Part model, mm, in its own coordinate system. A direction names the side the tool comes from. Give positions to 0.01 mm unless a question says otherwise; leave off trailing zeros. Write each loop counter-clockwise with the first axis right and the second up, starting at its lowest first coordinate (ties: lowest second). Pieces come first, ordered by that corner, then holes. Notation, with made-up numbers: M 74,-5.5 L 109,-5.5 A17 ccw 109,6.5 Z; hole C -11.5,-16 d6. An arc over 180 degrees is marked long. Use CSV: the item, a comma, the result in double quotes. Start each with the question number.
Item 1: Cut at B-B (z = 7). List the corners of the cut face in (x, y), then the cut area to 3 significant figures.
Item 2: Which spindle directions (+Z, -Z, +X, -X, +Y, -Y) get a long thin tool onto all of the face, cutting with end or side? Do faces 1 (the flat face through (0.8, 0, 0)), 2 (the flat face through (7, 0, 2.5)), 3 (the flat face through (5, -16, 2)), 4 (the cylindrical face through (5.042, 5.285, -0.051)), 5 (the cylindrical face through (1.877, 0.088, 0.528)). Say none if no direction does.
Item 3: Pin check, flat tips, straight feed: pin 1 (1.2 mm diameter, centred on x = 4.5, y = -8, fed in from -Z); pin 2 (0.6 mm diameter, centred on y = -13.5, z = 0, fed in from +X); pin 3 (1.2 mm diameter, centred on x = 3, y = 0.5, fed in from +Z). Stop position of each tip, or through.
Item 4: Cut at A-A (y = -21). List the corners of the cut face in (x, z), then the cut area to 3 significant figures.
Item 5: Cut at C-C (y = 0). List the corners of the cut face in (x, z) (3 decimals), then the cut area to 3 significant figures.
Item 6: Drill centre lines: line 1 (Z direction, x = 1.5, y = -10.5); line 2 (Y direction, x = 2, z = 5.25); line 3 (Y direction, x = 5, z = 0.5). Where is each one in solid material? Low to high. Write a range as [from, to].
Item 7: Cut at D-D (z = 3.5). List the corners of the cut face in (x, y), then the cut area to 3 significant figures.
Item 8: Mould opens along Y. For faces 6 (the flat face through (6, -15, 2)), 7 (the flat face through (2, 0, -2.5)), 8 (the flat face through (4.6, 16.4, 0.55)), 9 (the cylindrical face through (5.042, -4.699, -2.215)) say: released by +Y, released by -Y, zero draft, split by the parting line, or undercut.
from build123d import *

# Parameters (mm, degrees)
F0_W      = 58
F0_H      = 5
F1_DEPTH  = 2
F2_W      = 13
F2_H      = 0.5
F3_DEPTH  = 0.8
F4_W      = 58
F4_H      = 2.25
F5_DEPTH  = 6
F6_W      = 6
F6_H      = 10
F7_DEPTH  = 2.75
F8_R      = 2
F9_DEPTH  = 4
F10_R     = 1
F12_DEPTH = 4
F13_W     = 22
F13_H     = 5
F14_DEPTH = 0.8
F15_R     = 0.5
F16_W     = 6.8
F16_H     = 13
F17_DEPTH = 0.3
F18_W     = 3
F18_H     = 3
F19_DEPTH = 1.95


# Not quite as in the source:
# - a pattern or mirror of a feature is missing from the dataset's text; its kind, count and spacing are read off the source's solid


with BuildPart() as f1:
    # F0 (on Right) → F1 (new body)
    with BuildSketch(Plane.YZ):
        Rectangle(F0_W, F0_H)
    extrude(amount=F1_DEPTH)

    # F2 (on face) → F3 (cut)
    with BuildSketch(Plane.YZ.offset(2)):
        with Locations((16.5, 0)):
            Rectangle(F2_W, F2_H)
        with Locations((-16.5, 0)):
            Rectangle(F2_W, F2_H)
    extrude(amount=-F3_DEPTH, mode=Mode.SUBTRACT)

    # F4 (on face) → F5 (join)
    with BuildSketch(Plane.YZ.offset(2)):
        with Locations((0, 1.375)):
            Rectangle(F4_W, F4_H)
    extrude(amount=F5_DEPTH)

    # F6 (on face) → F7 (join, through all)
    with BuildSketch(Plane(origin=(0, 0, 0.25), x_dir=(1, 0, 0), z_dir=(0, 0, -1))):
        with Locations((5, 0)):
            Rectangle(F6_W, F6_H)
    extrude(amount=F7_DEPTH)

    # F8 (on face) → F9 (cut)
    with BuildSketch(Plane.XY.offset(2.5)):
        with Locations((3.875, 0)):
            Circle(F8_R)
    extrude(amount=-F9_DEPTH, mode=Mode.SUBTRACT)

    # F10
    f10_edges = [f1.edges().sort_by_distance(p)[0] for p in [
        (5, -5, -2.5),
        (5, -5, 0.25),
        (5, 5, 0.25),
        (5, 5, -2.5),
    ]]
    fillet(f10_edges, radius=F10_R)

    # F11 (on face) → F12 (join)
    with BuildSketch(Plane(origin=(0, 29, 0), x_dir=(-1, 0, 0), z_dir=(0, 1, 0))):
        Polygon((-4, 2.5), (0, 2.5), (0, 9), (-2, 9), align=None)
    f12 = extrude(amount=-F12_DEPTH)

    # F12_copies: F12 across plane
    add(f12.mirror(Plane(origin=(0, 0, 0), x_dir=(0, 0, -1), z_dir=(0, -1, 0))))

    # F13 (on face) → F14 (cut)
    with BuildSketch(Plane(origin=(0, 0, 0), x_dir=(0, -1, 0), z_dir=(-1, 0, 0))):
        Rectangle(F13_W, F13_H)
    extrude(amount=-F14_DEPTH, mode=Mode.SUBTRACT)

    # F15
    f15_edges = [f1.edges().sort_by_distance(p)[0] for p in [
        (0.8, 11, 0),
        (0.8, -11, 0),
        (4, 27, 2.5),
        (2, 25, 2.5),
        (2, -25, 2.5),
        (4, -27, 2.5),
    ]]
    fillet(f15_edges, radius=F15_R)

    # F16 (on face) → F17 (cut)
    with BuildSketch(Plane(origin=(0, 0, 0.25), x_dir=(1, 0, 0), z_dir=(0, 0, -1))):
        with Locations((4.6, 16.5)):
            Rectangle(F16_W, F16_H)
        with Locations((4.6, -16.5)):
            Rectangle(F16_W, F16_H)
    extrude(amount=-F17_DEPTH, mode=Mode.SUBTRACT)

    # F18 (on face) → F19 (cut, through all)
    with BuildSketch(Plane(origin=(0, 0, 0.55), x_dir=(1, 0, 0), z_dir=(0, 0, -1))):
        with Locations((6.5, -16.5)):
            Rectangle(F18_W, F18_H)
        with Locations((6.5, 16.5)):
            Rectangle(F18_W, F18_H)
    extrude(amount=-F19_DEPTH, mode=Mode.SUBTRACT)


solid = f1.part
Worked answers:
1,outline,"M 0,-29 L 2.62,-29 L 2.62,-25 L 0,-25 Z; M 0,25 L 2.62,25 L 2.62,29 L 0,29 Z"
1,area,"20.9 mm^2"
2,face 1,"+Z, -Z, -X"
2,face 2,"+Z, +X"
2,face 3,"+Z, -Z, +X"
2,face 4,"-Z, +X, +Y"
2,face 5,"+Z"
3,pin 1,"stops at z = 0.25"
3,pin 2,"stops at x = 2"
3,pin 3,"stops at z = -1.5"
4,outline,"M 0,-2.5 L 2,-2.5 L 2,-0.25 L 1.2,-0.25 L 1.2,0.55 L 8,0.55 L 8,2.5 L 0,2.5 Z"
4,area,"21.1 mm^2"
5,outline,"M 0.8,-2.5 L 8,-2.5 L 8,2.5 L 5.875,2.5 L 5.875,-1.5 L 1.875,-1.5 L 1.875,2.5 L 0.8,2.5 Z"
5,area,"20.0 mm^2"
6,line 1,"z = [-2.5, -0.25], [0.55, 2.5]"
6,line 2,"y = [-29, -25], [25, 29]"
6,line 3,"y = [-29, -23], [-10, -1.65], [1.65, 10], [23, 29]"
7,outline,"M 0,-29 L 3.69,-29 L 3.69,-25 L 0,-25 Z; M 0,25 L 3.69,25 L 3.69,29 L 0,29 Z"
7,area,"29.5 mm^2"
8,face 6,"undercut"
8,face 7,"zero draft"
8,face 8,"undercut"
8,face 9,"released by -Y"
